```python
from build123d import *

# Parameters (mm, degrees)
SKETCH1_R           = 47.5
BOSS_EXTRUDE1_DEPTH = 4.5


with BuildPart() as part:
    # Sketch1 → Boss-Extrude1 (new body, symmetric)
    with BuildSketch(Plane.XY):
        with BuildLine():
            Line((250, -99.41125497), (250, -60.550262484))
            ThreePointArc((250, -60.550262484), (247.071067812, -53.479194672), (240, -50.550262484))
            Line((240, -50.550262484), (211.253965719, -50.550262484))
            Line((211.253965719, -50.550262484), (211.253965719, 85.284392818))
            Line((211.253965719, 85.284392818), (112.411473654, 184.126884883))
            Line((112.411473654, 184.126884883), (133.84792187, 205.563333099))
            ThreePointArc((133.84792187, 205.563333099), (136.776854058, 212.634400911), (133.84792187, 219.705468723))
            Line((133.84792187, 219.705468723), (106.482322781, 247.071067812))
            ThreePointArc((106.482322781, 247.071067812), (103.238089293, 249.238795325), (99.41125497, 250))
            Line((99.41125497, 250), (-99.41125497, 250))
            ThreePointArc((-99.41125497, 250), (-103.238089293, 249.238795325), (-106.482322781, 247.071067812))
            Line((-106.482322781, 247.071067812), (-247.071067812, 106.482322781))
            ThreePointArc((-247.071067812, 106.482322781), (-249.238795325, 103.238089293), (-250, 99.41125497))
            Line((-250, 99.41125497), (-250, -99.41125497))
            ThreePointArc((-250, -99.41125497), (-249.238795325, -103.238089293), (-247.071067812, -106.482322781))
            Line((-247.071067812, -106.482322781), (-103.553390593, -250))
            Line((-103.553390593, -250), (103.553390593, -250))
            Line((103.553390593, -250), (247.071067812, -106.482322781))
            ThreePointArc((247.071067812, -106.482322781), (249.238795325, -103.238089293), (250, -99.41125497))
        make_face()
        with Locations((0, 135.632011386)):
            Circle(SKETCH1_R, mode=Mode.SUBTRACT)
        with BuildLine():
            Line((-200, 54.5), (-191, 54.5))
            ThreePointArc((-191, 54.5), (-187.82, 51.32), (-191, 48.14))
            Line((-191, 48.14), (-191, -48.14))
            ThreePointArc((-191, -48.14), (-187.82, -51.32), (-191, -54.5))
            Line((-191, -54.5), (-200, -54.5))
            ThreePointArc((-200, -54.5), (-203.18, -51.32), (-200, -48.14))
            Line((-200, -48.14), (-200, 48.14))
            ThreePointArc((-200, 48.14), (-203.18, 51.32), (-200, 54.5))
        make_face(mode=Mode.SUBTRACT)
        with BuildLine():
            Line((-105.811554275, 183.200760604), (-173.891795168, 115.120519711))
            ThreePointArc((-173.891795168, 115.120519711), (-178.388994296, 115.120519711), (-178.388994296, 110.623320583))
            Line((-178.388994296, 110.623320583), (-172.025033265, 104.259359552))
            ThreePointArc((-172.025033265, 104.259359552), (-167.527834137, 104.259359552), (-167.527834137, 108.756558681))
            Line((-167.527834137, 108.756558681), (-99.447593244, 176.836799573))
            ThreePointArc((-99.447593244, 176.836799573), (-94.950394116, 176.836799573), (-94.950394116, 181.333998701))
            Line((-94.950394116, 181.333998701), (-101.314355147, 187.697959732))
            ThreePointArc((-101.314355147, 187.697959732), (-105.811554275, 187.697959732), (-105.811554275, 183.200760604))
        make_face(mode=Mode.SUBTRACT)
        with BuildLine():
            Line((56.292114102, 212.101851618), (-39.987885898, 212.101851618))
            ThreePointArc((-39.987885898, 212.101851618), (-43.167885898, 215.281851618), (-46.347885898, 212.101851618))
            Line((-46.347885898, 212.101851618), (-46.347885898, 203.101851618))
            ThreePointArc((-46.347885898, 203.101851618), (-43.167885898, 199.921851618), (-39.987885898, 203.101851618))
            Line((-39.987885898, 203.101851618), (56.292114102, 203.101851618))
            ThreePointArc((56.292114102, 203.101851618), (59.472114102, 199.921851618), (62.652114102, 203.101851618))
            Line((62.652114102, 203.101851618), (62.652114102, 212.101851618))
            ThreePointArc((62.652114102, 212.101851618), (59.472114102, 215.281851618), (56.292114102, 212.101851618))
        make_face(mode=Mode.SUBTRACT)
        with BuildLine():
            Line((126.065519994, -179.251023088), (194.145760887, -111.170782195))
            ThreePointArc((194.145760887, -111.170782195), (198.642960015, -111.170782195), (198.642960015, -106.673583067))
            Line((198.642960015, -106.673583067), (192.278998984, -100.309622036))
            ThreePointArc((192.278998984, -100.309622036), (187.781799856, -100.309622036), (187.781799856, -104.806821165))
            Line((187.781799856, -104.806821165), (119.701558963, -172.887062057))
            ThreePointArc((119.701558963, -172.887062057), (115.204359835, -172.887062057), (115.204359835, -177.384261185))
            Line((115.204359835, -177.384261185), (121.568320866, -183.748222216))
            ThreePointArc((121.568320866, -183.748222216), (126.065519994, -183.748222216), (126.065519994, -179.251023088))
        make_face(mode=Mode.SUBTRACT)
        with BuildLine():
            Line((-36.038148382, -208.152114102), (60.241851618, -208.152114102))
            ThreePointArc((60.241851618, -208.152114102), (63.421851618, -211.332114102), (66.601851618, -208.152114102))
            Line((66.601851618, -208.152114102), (66.601851618, -199.152114102))
            ThreePointArc((66.601851618, -199.152114102), (63.421851618, -195.972114102), (60.241851618, -199.152114102))
            Line((60.241851618, -199.152114102), (-36.038148382, -199.152114102))
            ThreePointArc((-36.038148382, -199.152114102), (-39.218148382, -195.972114102), (-42.398148382, -199.152114102))
            Line((-42.398148382, -199.152114102), (-42.398148382, -208.152114102))
            ThreePointArc((-42.398148382, -208.152114102), (-39.218148382, -211.332114102), (-36.038148382, -208.152114102))
        make_face(mode=Mode.SUBTRACT)
        with BuildLine():
            Line((-171.098908986, -113.963668377), (-103.018668094, -182.043909269))
            ThreePointArc((-103.018668094, -182.043909269), (-103.018668094, -186.541108398), (-98.521468965, -186.541108398))
            Line((-98.521468965, -186.541108398), (-92.157507935, -180.177147367))
            ThreePointArc((-92.157507935, -180.177147367), (-92.157507935, -175.679948239), (-96.654707063, -175.679948239))
            Line((-96.654707063, -175.679948239), (-164.734947956, -107.599707346))
            ThreePointArc((-164.734947956, -107.599707346), (-164.734947956, -103.102508218), (-169.232147084, -103.102508218))
            Line((-169.232147084, -103.102508218), (-175.596108115, -109.466469248))
            ThreePointArc((-175.596108115, -109.466469248), (-175.596108115, -113.963668377), (-171.098908986, -113.963668377))
        make_face(mode=Mode.SUBTRACT)
        with BuildLine():
            Line((-134, -88.91125497), (-66, -88.91125497))
            ThreePointArc((-66, -88.91125497), (-63, -91.91125497), (-60, -88.91125497))
            Line((-60, -88.91125497), (-60, -79.91125497))
            ThreePointArc((-60, -79.91125497), (-63, -76.91125497), (-66, -79.91125497))
            Line((-66, -79.91125497), (-134, -79.91125497))
            ThreePointArc((-134, -79.91125497), (-137, -76.91125497), (-140, -79.91125497))
            Line((-140, -79.91125497), (-140, -88.91125497))
            ThreePointArc((-140, -88.91125497), (-137, -91.91125497), (-134, -88.91125497))
        make_face(mode=Mode.SUBTRACT)
        with BuildLine():
            Line((140, -88.91125497), (140, -79.91125497))
            ThreePointArc((140, -79.91125497), (137, -76.91125497), (134, -79.91125497))
            Line((134, -79.91125497), (66, -79.91125497))
            ThreePointArc((66, -79.91125497), (63, -76.91125497), (60, -79.91125497))
            Line((60, -79.91125497), (60, -88.91125497))
            ThreePointArc((60, -88.91125497), (63, -91.91125497), (66, -88.91125497))
            Line((66, -88.91125497), (134, -88.91125497))
            ThreePointArc((134, -88.91125497), (137, -91.91125497), (140, -88.91125497))
        make_face(mode=Mode.SUBTRACT)
    extrude(amount=BOSS_EXTRUDE1_DEPTH, both=True)


solid = part.part
```
Check sheet for the modelled part. Datum: model origin and axes. Units: mm. A direction names the side the tool comes from. Round coordinates to 2 decimals unless told otherwise and drop trailing zeros. Loops run counter-clockwise (first coordinate to the right, second up) from the corner with the lowest first, then second, coordinate; pieces in that order, holes last. Notation, with made-up numbers: (31.5, -14) -> (57.5, -14) arc R30 cw to (57.5, 19) -> close; hole circle Ø4 at (38.5, 82). An arc over 180 degrees is marked (long way). Write item = value, one per line. Start each with the question number.
1) Sectioned sample at C-C, the plane x = 170. Record the cut outline in (y, z).
2) Sectioned sample at D-D, the plane z = 0.25. State how many separate pieces and enclosed holes the cut face has, plus the area to 3 significant figures.
3) Set-up check for faces 1 (the flat face through (-130.218, -142.116, 0.063)), 2 (the flat face through (162.525, 134.014, 0.063)), 3 (the flat face through (-175.793, 177.761, 0.063)): record each of +Z, -Z, +X, -X, +Y, -Y from which the full face is reachable in a straight line by a thin tool's end or side.
4) Gauge pin test, flat ends, axial feed: pin 1 Ø4.5 at (x, z) = (232, -2) entering from +Y; pin 2 Ø4.5 at (y, z) = (4, 0) entering from +X; pin 3 Ø2.5 at (x, z) = (-196, -2) entering from -Y. Record the tip position at first contact, or that the pin passes through.
5) Sectioned sample at A-A, the plane x = 0. Record the cut outline in (y, z), plus the area to 3 significant figures.
6) Thickness scan on probe 1 along Y at (x, z) = (0, 1.75); probe 2 along X at (y, z) = (-81.5, -3.75); probe 3 along Y at (x, z) = (54, 1.25). Record the ranges inside material, lowest first.
7) Sectioned sample at B-B, the plane y = 3. Record the cut outline in (x, z), plus the area to 3 significant figures.
8) Release check for a two-part mould opening along Y. For faces 4 (the flat face through (154.22, -138.37, 0.06)), 5 (the flat face through (174.308, -179.246, 0.063)), 6 (the flat face through (-3, 3, 4.5)) record: released by +Y, released by -Y, zero draft, split by the parting line, or undercut.
Results are:
q1.outline = (-183.55, -4.5) -> (-135.32, -4.5) -> (-135.32, 4.5) -> (-183.55, 4.5) -> close; (-122.59, -4.5) -> (126.54, -4.5) -> (126.54, 4.5) -> (-122.59, 4.5) -> close
q2.separate_pieces = 1
q2.enclosed_holes = 9
q2.area = 181,000 mm^2
q3.face_1 = +Z, -Z
q3.face_2 = +Z, -Z, +X
q3.face_3 = +Z, -Z, -X, +Y
q4.pin_1 = -50.55
q4.pin_2 = 211.25
q4.pin_3 = -158.8
q5.outline = (-250, -4.5) -> (-208.15, -4.5) -> (-208.15, 4.5) -> (-250, 4.5) -> close; (-199.15, -4.5) -> (88.13, -4.5) -> (88.13, 4.5) -> (-199.15, 4.5) -> close; (183.13, -4.5) -> (203.1, -4.5) -> (203.1, 4.5) -> (183.13, 4.5) -> close; (212.1, -4.5) -> (250, -4.5) -> (250, 4.5) -> (212.1, 4.5) -> close
q5.area = 3,480 mm^2
q6.probe_1 = -250 to -208.15, -199.15 to 88.13, 183.13 to 203.1, 212.1 to 250
q6.probe_2 = -250 to -140, -60 to 60, 140 to 250
q6.probe_3 = -250 to -208.15, -199.15 to 203.1, 212.1 to 250
q7.outline = (-250, -4.5) -> (-200, -4.5) -> (-200, 4.5) -> (-250, 4.5) -> close; (-191, -4.5) -> (211.25, -4.5) -> (211.25, 4.5) -> (-191, 4.5) -> close
q7.area = 4,070 mm^2
q8.face_4 = undercut
q8.face_5 = released by -Y
q8.face_6 = zero draft
